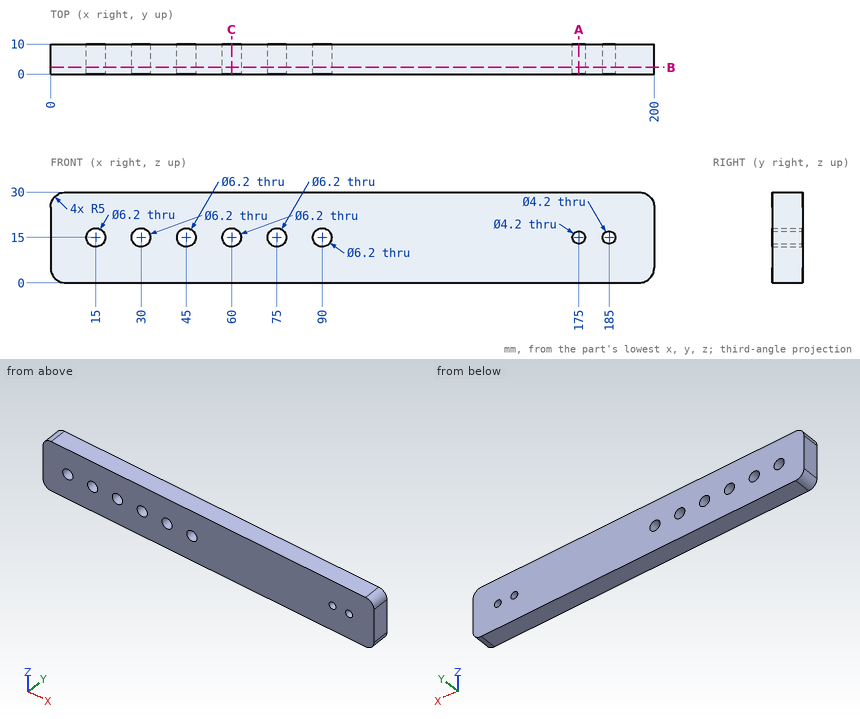
Verification items for this drawing (mm, ordinates from the low corner). Give positions to 0.01 mm unless a question says otherwise; leave off trailing zeros. Loops run counter-clockwise (first coordinate to the right, second up) from the corner with the lowest first, then second, coordinate; pieces in that order, holes last. Notation, with made-up numbers: M 19,-6 L 77,-6 A14 ccw 77,9 Z; hole C -39.75,-17.75 d6. An arc over 180 degrees is marked long. Return JSON: item names as keys, results as strings. Group by question number.
1. Cross-section at C-C on x = 60. Record the boundary of the cut face in (y, z), plus the area to 3 significant figures.
2. Cross-section at A-A on x = 175. Record the boundary of the cut face in (y, z), plus the area to 3 significant figures.
3. Cross-section at B-B on y = 2.25. State how many separate pieces and enclosed holes the cut face has, plus the area to 3 significant figures.
4. Thickness scan on L1, parallel to Z at x = 185, y = 7; L2, parallel to Z at x = 30, y = 2.25; L3, parallel to X at y = 3.5, z = 3.5. Record the ranges inside material, lowest first.
Return value:
{
 "1": {"outline": "M 0,0 L 10,0 L 10,11.9 L 0,11.9 Z; M 0,18.1 L 10,18.1 L 10,30 L 0,30 Z", "area": "238 mm^2"},
 "2": {"outline": "M 0,0 L 10,0 L 10,12.9 L 0,12.9 Z; M 0,17.1 L 10,17.1 L 10,30 L 0,30 Z", "area": "258 mm^2"},
 "3": {"separate pieces": "1", "enclosed holes": "8", "area": "5,770 mm^2"},
 "4": {"L1": "0 to 12.9, 17.1 to 30", "L2": "0 to 11.9, 18.1 to 30", "L3": "0.23 to 199.77"}
}
